from build123d import *

# Parameters (mm, degrees)
SKETCH001_R     = 10.612882
POCKET_DEPTH    = 4.001
SKETCH002_R     = 5
POCKET001_DEPTH = 4.001
CHAMFER_SIZE    = 0.5


with BuildPart() as part:
    # Sketch → Revolution (revolve)
    with BuildSketch(Plane.XZ):
        Polygon((0, 4), (8.25, 4), (9.6, 3.220577), (9.6, 0.779423), (8.25, 0), (0, 0), align=None)
    revolve(axis=Axis((0, 0, 0), (0, 0, 1)))

    # Sketch001 → Pocket (cut, through all)
    with BuildSketch(Plane(origin=(0, 0, 4), x_dir=(-1, 0, 0), z_dir=(0, 0, 1))):
        Circle(SKETCH001_R)
        Polygon((-8.325, 4.806441), (0, 9.612882), (8.325, 4.806441), (8.325, -4.806441), (0, -9.612882), (-8.325, -4.806441), align=None, mode=Mode.SUBTRACT)
    extrude(amount=-POCKET_DEPTH, mode=Mode.SUBTRACT)

    # Sketch002 → Pocket001 (cut, through all)
    with BuildSketch(Plane(origin=(0, 0, 4), x_dir=(-1, 0, 0), z_dir=(0, 0, 1))):
        with Locations((0.036806, -0.027604)):
            Circle(SKETCH002_R)
    extrude(amount=-POCKET001_DEPTH, mode=Mode.SUBTRACT)

    # Chamfer
    chamfer_edges = [part.edges().sort_by_distance(p)[0] for p in [
        (4.963194, 0.027604, 4),
        (4.963194, 0.027604, 0),
    ]]
    chamfer(chamfer_edges, length=CHAMFER_SIZE)


solid = part.part
Work out the finished part from the listing and answer in its coordinate system (mm). Round coordinates to 2 decimals unless told otherwise and drop trailing zeros. One line per item, written item: value.
Q1. Straight lines are drawn through the part: line 1 (X direction, y = 0, z = 1.3) (3 decimals); line 2 (X direction, y = 4, z = 3.8); line 3 (Y direction, x = 1.5, z = 1.35). For each, find the intervals that lie inside material, in ascending order.
Derived:
line 1: -8.325 to -5.037, 4.963 to 8.325
line 2: -7.61 to -3.55, 3.47 to 7.61
line 3: -8.75 to -4.73, 4.79 to 8.75
Q2. Determine the mould class of faces 1 (the face through (8.325, 0, 2)), 2 (the face through (4.105, 7.243, 2.027)), 3 (the face through (1.05, 4.91, 2.02)) for opening direction Y: released by +Y, released by -Y, zero draft, split by the parting line, or undercut.
Derived:
face 1: zero draft
face 2: released by +Y
face 3: undercut
Q3. Flat-ended cylindrical pins translate along their axes: pin 1 (1.5 mm diameter, centred on x = -6.5, y = -6.5, fed in from -Z); pin 2 (1 mm diameter, centred on y = 6.5, z = 3, fed in from +X); pin 3 (1 mm diameter, centred on x = -4, z = 0.5, fed in from -Y). Find the tip coordinate at first contact, or state that the pin passes through.
Derived:
pin 1: z = 0.11
pin 2: x = 6.26
pin 3: y = -7.59
